Check sheet for the modelled part. Datum: model origin and axes. Units: mm. A direction names the side the tool comes from. Coordinates: 2 decimals unless noted, no trailing zeros. Order: outer loops, then holes, each group sorted by start corner. A loop starts at its lowest first (then second) coordinate and runs counter-clockwise, first axis right, second up. Notation, with made-up numbers: M 9,-21 L 43,-21 A19 ccw 43,-1 Z; hole C 81.5,84 d9. An arc over 180 degrees is marked long. Answer in a Markdown table with one row per item. Add a question column.
from build123d import *

# Parameters (mm, degrees)
SKETCH091_R     = 4
PAD034_DEPTH    = 28
SKETCH092_R     = 6.5
PAD035_DEPTH    = 8
POCKET034_DEPTH = 5


with BuildPart() as part:
    # Sketch091 → Pad034 (new body)
    with BuildSketch(Plane.YZ):
        Circle(SKETCH091_R)
    extrude(amount=PAD034_DEPTH)

    # Sketch092 → Pad035 (join)
    with BuildSketch(Plane.YZ):
        Circle(SKETCH092_R)
    extrude(amount=PAD035_DEPTH)

    # Sketch093 → Pocket034 (cut)
    with BuildSketch(Plane.YZ):
        Polygon((3, 1.732051), (0, 3.464102), (-3, 1.732051), (-3, -1.732051), (0, -3.464102), (3, -1.732051), align=None)
    extrude(amount=POCKET034_DEPTH, mode=Mode.SUBTRACT)


with BuildPart() as part_1:
    # Body020 placement: moved
    add(part.part.moved(Location((19.600528, -17, -16.6))))


solid = part_1.part
1. Release check for a two-part mould opening along Y. For faces 4 (the cylindrical face through (23.545, -22.158, -20.555)), 5 (the flat face through (22.1, -18.5, -14)), 6 (the flat face through (47.601, -17, -17)) record: released by +Y, released by -Y, zero draft, split by the parting line, or undercut.
2. Section check A-A on x = 22.25. Enter the section's corners in (y, z), then the cut area to 3 significant figures.
3. Set-up check for faces 1 (the cylindrical face through (37.5, -20.2, -19)), 2 (the flat face through (19.601, -18.5, -19.4)), 3 (the flat face through (22.1, -18.5, -19.2)): record each of +Z, -Z, +X, -X, +Y, -Y from which the full face is reachable in a straight line by a thin tool's end or side.
4. Section check B-B on z = -16.6. Enter the section's corners in (x, y), then the cut area to 3 significant figures.
5. Section check D-D on x = 31.75. Enter the section's corners in (y, z), then the cut area to 3 significant figures.
6. Go/stop test with flat-tipped pins: pin 1 Ø1 at (x, y) = (40, -15) entering from -Z; pin 2 Ø5 at (x, z) = (25, -17) entering from -Y; pin 3 Ø1.5 at (x, y) = (29.5, -15) entering from -Z; pin 4 Ø5 at (x, z) = (36, -11.5) entering from -Y. Record where each tip stops, or that it passes through.
7. Section check C-C on y = -17.75. Enter the section's corners in (x, z).
8. Scan lines: line 1 (X direction, y = -22.25, z = -17); line 2 (Y direction, x = 42.75, z = -16.75); line 3 (Z direction, x = 28.5, y = -18.5). Record each from-to range of solid material in increasing order.
Result sheet:
| question | item | result |
|---|---|---|
| 1 | face 4 | split by the parting line |
| 1 | face 5 | undercut |
| 1 | face 6 | zero draft |
| 2 | outline | C -17,-16.6 d13; hole M -20,-18.33 L -17,-20.06 L -14,-18.33 L -14,-14.87 L -17,-13.14 L -20,-14.87 Z |
| 2 | area | 102 mm^2 |
| 3 | face 1 | +X |
| 3 | face 2 | +Z, -Z, -X, +Y, -Y |
| 3 | face 3 | -X |
| 4 | outline | M 19.6,-23.5 L 27.6,-23.5 L 27.6,-21 L 47.6,-21 L 47.6,-13 L 27.6,-13 L 27.6,-10.5 L 19.6,-10.5 L 19.6,-14 L 24.6,-14 L 24.6,-20 L 19.6,-20 Z |
| 4 | area | 234 mm^2 |
| 5 | outline | C -17,-16.6 d8 |
| 5 | area | 50.3 mm^2 |
| 6 | pin 1 | z = -20.31 |
| 6 | pin 2 | y = -23.5 |
| 6 | pin 3 | z = -20.4 |
| 6 | pin 4 | y = -20.04 |
| 7 | outline | M 19.6,-23.06 L 27.6,-23.06 L 27.6,-20.53 L 47.6,-20.53 L 47.6,-12.67 L 27.6,-12.67 L 27.6,-10.14 L 19.6,-10.14 L 19.6,-13.57 L 24.6,-13.57 L 24.6,-19.63 L 19.6,-19.63 Z |
| 8 | line 1 | 19.6 to 27.6 |
| 8 | line 2 | -21 to -13 |
| 8 | line 3 | -20.31 to -12.89 |
